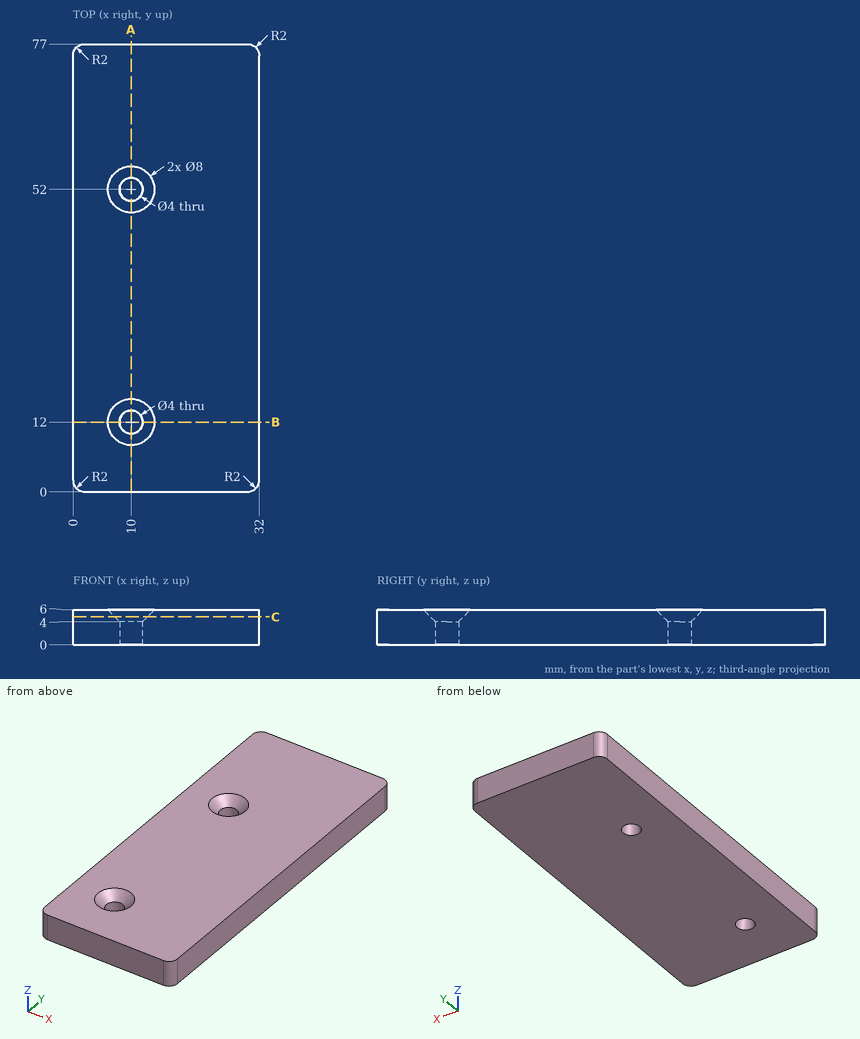
Could you check a few things on this drawing? It's one solid part, dimensions in mm from its lowest x, y, z. Round coordinates to 2 decimals unless told otherwise and drop trailing zeros. Order: outer loops, then holes, each group sorted by start corner. A loop starts at its lowest first (then second) coordinate and runs counter-clockwise, first axis right, second up. Notation, with made-up numbers: M 17,8.25 L 48,8.25 A7 cw 48,16.25 Z; hole C 66,7.5 d7. An arc over 180 degrees is marked long. One line per item, written item: value.
(1) I'm going to push a flat-ended pin straight in: P1, Ø3.5, axis at x = 10, y = 12, coming from the -Z side. Where does the tip first touch, or does it pass through?
Ans:
P1: passes through
(2) Imagine slicing it at A-A (x = 10). Write out the boundary of the cut face in (y, z), and give its area (3 significant figures).
Ans:
outline: M 0,0 L 10,0 L 10,4 L 8,6 L 0,6 Z; M 14,0 L 50,0 L 50,4 L 48,6 L 16,6 L 14,4 Z; M 54,0 L 77,0 L 77,6 L 56,6 L 54,4 Z
area: 406 mm^2
(3) I need wall thicknesses on line 1 along Y through (x, z) = (10, 2.4); line 2 along X through (y, z) = (12, 1.2). Which ranges of each line are inside material? Lowest first, please. Write a range as from..to.
Ans:
line 1: y = 0..10, 14..50, 54..77
line 2: x = 0..8, 12..32
(4) Imagine slicing it at B-B (y = 12). Write out the boundary of the cut face in (x, z).
Ans:
outline: M 0,0 L 8,0 L 8,4 L 6,6 L 0,6 Z; M 12,0 L 32,0 L 32,6 L 14,6 L 12,4 Z
(5) Imagine slicing it at C-C (z = 4.8). Write out the boundary of the cut face in (x, y), and give its area (3 significant figures).
Ans:
outline: M 0,2 A2 ccw 2,0 L 30,0 A2 ccw 32,2 L 32,75 A2 ccw 30,77 L 2,77 A2 ccw 0,75 Z; hole C 10,12 d5.6; hole C 10,52 d5.6
area: 2,410 mm^2
